Can you work these out from the model? Positions are in its coordinate system, mm. Coordinates: 2 decimals unless noted, no trailing zeros. Order: outer loops, then holes, each group sorted by start corner. A loop starts at its lowest first (then second) coordinate and runs counter-clockwise, first axis right, second up. Notation, with made-up numbers: (-0.75, 64.5) -> (31.25, 64.5) arc R36 ccw to (31.25, 100.5) -> close; hole circle Ø6 at (-37, 57). An arc over 180 degrees is marked (long way). Answer as a JSON object with one key per item and string values. Group by question number.
(1) I want a section at B-B, the plane x = 1. List the corners of the cut face in (y, z) for me.
(2) I need wall thicknesses on line 1 (X direction, y = -3.5, z = -0.5); line 2 (Y direction, x = 80, z = -2.5); line 3 (X direction, y = -4.25, z = -6.75). Which ranges of each line are inside material? Lowest first, please.
(3) I want a section at D-D, the plane y = 7.5. List the corners of the cut face in (x, z) for me.
(4) For pin 1 (1.5 mm diameter, centred on y = 1, z = -1.5, fed in from -X); pin 2 (4 mm diameter, centred on y = -7.5, z = -2.5, fed in from -X); pin 3 (1 mm diameter, centred on y = 3.5, z = -3.5, fed in from +X), each with a flat end and sliding along its axis, tell me the tip position at first contact or that it passes through.
(5) I want a section at C-C, the plane z = -4. List the corners of the cut face in (x, y) for me, plus the area to 3 significant figures.
(6) I want a section at A-A, the plane y = 0. List the corners of the cut face in (x, z) for me.
(7) If we mould it in two halves opening along X, with no side actions, what happens to faces 1 (the flat face through (41, 10, -5)), 2 (the cylindrical face through (-10, 0, -5)), 3 (the cylindrical face through (-1.08, -4.88, -4.93))? For each: pulls with the +X half, pulls with the -X half, needs draft (parallel to the pull), parting line crosses it, or undercut.
from build123d import *

# Parameters (mm, degrees)
F1_DEPTH = 10
F2_R     = 5
F3_DEPTH = 10.001


with BuildPart() as f1:
    # F0 (on Top) → F1 (new body)
    with BuildSketch(Plane.XY):
        with BuildLine():
            Line((80, 10), (0, 10))
            ThreePointArc((0, 10), (-10, 0), (0, -10))
            Line((0, -10), (80, -10))
            ThreePointArc((80, -10), (90, 0), (80, 10))
        make_face()
    extrude(amount=-F1_DEPTH)

    # F2 (on face) → F3 (cut, through all)
    with BuildSketch(Plane.XY):
        Circle(F2_R)
        with Locations((80, 0)):
            Circle(F2_R)
    extrude(amount=-F3_DEPTH, mode=Mode.SUBTRACT)


solid = f1.part
Computed values:
{
 "1": {"outline": "(-10, -10) -> (-4.9, -10) -> (-4.9, 0) -> (-10, 0) -> close; (4.9, -10) -> (10, -10) -> (10, 0) -> (4.9, 0) -> close"},
 "2": {"line 1": "x = -9.37 to -3.57, 3.57 to 76.43, 83.57 to 89.37", "line 2": "y = -10 to -5, 5 to 10", "line 3": "x = -9.05 to -2.63, 2.63 to 77.37, 82.63 to 89.05"},
 "3": {"outline": "(-6.61, -10) -> (86.61, -10) -> (86.61, 0) -> (-6.61, 0) -> close"},
 "4": {"pin 1": "stops at x = -10", "pin 2": "stops at x = -8.35", "pin 3": "stops at x = 89.54"},
 "5": {"outline": "(0, -10) -> (80, -10) arc R10 ccw to (80, 10) -> (0, 10) arc R10 ccw to start; hole circle Ø10 at (0, 0); hole circle Ø10 at (80, 0)", "area": "1,760 mm2"},
 "6": {"outline": "(-10, -10) -> (-5, -10) -> (-5, 0) -> (-10, 0) -> close; (5, -10) -> (75, -10) -> (75, 0) -> (5, 0) -> close; (85, -10) -> (90, -10) -> (90, 0) -> (85, 0) -> close"},
 "7": {"face 1": "needs draft", "face 2": "pulls with the -X half", "face 3": "undercut"}
}
